```python
from build123d import *

# Parameters (mm, degrees)
F1_DEPTH  = 127
F2_R      = 104.325393
F2_R_2    = 26.179728
F2_R_3    = 10.594913
F3_DEPTH  = 38.1
F3_FACE_R = 10.594913
F4_DEPTH  = 38.1
F5_R      = 9.525
F6_DEPTH  = 127


with BuildPart() as f1:
    # F0 (on Front) → F1 (new body)
    with BuildSketch(Plane.XZ):
        Polygon((12.158688, 37.641967), (-25.941312, 37.641967), (-25.941312, -13.158033), (-16.416312, -13.158033), (-16.416312, -25.858033), (2.62328, -25.858033), (2.62328, -13.26213), (12.158688, -13.26213), align=None)
    extrude(amount=F1_DEPTH)

    # F2 (on Right) → F3 (cut)
    with BuildSketch(Plane.YZ):
        with Locations((-442.556002, 14.38355)):
            Circle(F2_R)
        with Locations((196.325033, 10.431935)):
            Circle(F2_R_2)
        with Locations((-94.180087, 11.172054)):
            Circle(F2_R_3)
        with Locations((-32.819913, 11.172054)):
            Circle(F2_R_3)
    extrude(amount=-F3_DEPTH, mode=Mode.SUBTRACT)

    # F3_face (on face) → F4 (cut)
    with BuildSketch(Plane(origin=(0, -32.819913, 11.172054), x_dir=(0, 1, 0), z_dir=(-1, 0, 0))):
        Circle(F3_FACE_R)
        with Locations((-61.360174, 0)):
            Circle(F3_FACE_R)
    extrude(amount=-F4_DEPTH, mode=Mode.SUBTRACT)

    # F5 (on Front) → F6 (cut)
    with BuildSketch(Plane.XZ):
        with Locations((-6.891312, 12.241967)):
            Circle(F5_R)
    extrude(amount=F6_DEPTH, mode=Mode.SUBTRACT)


solid = f1.part
```
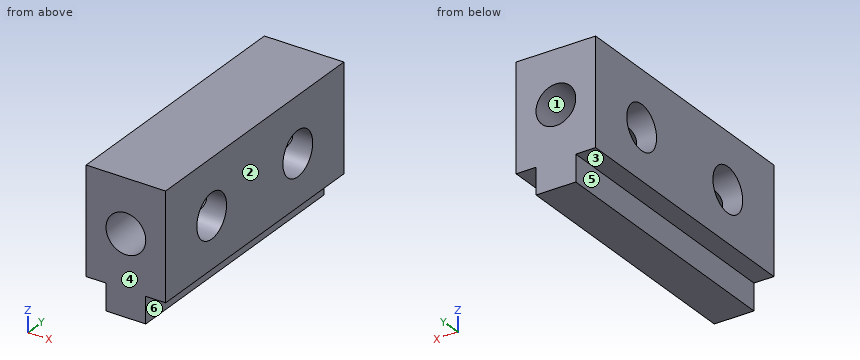
Geometry check sheet. Reference: the model listing, model coordinates, mm. Face numbers are marked on the shaded views. A direction names the side the tool comes from. Coordinates: 2 decimals unless noted, no trailing zeros. Write each loop counter-clockwise with the first axis right and the second up, starting at its lowest first coordinate (ties: lowest second). Pieces come first, ordered by that corner, then holes. Notation, with made-up numbers: (57, 36) -> (89, 36) arc R9 cw to (89, 46) -> close; hole circle Ø2 at (75.25, 85.5). An arc over 180 degrees is marked (long way). Use CSV: the item, a comma, the result in double quotes. Start each with the question number.
Item 1: Set-up check for the marked faces 4, 5 and 6: record each of +Z, -Z, +X, -X, +Y, -Y from which the full face is reachable in a straight line by a thin tool's end or side.
Item 2: Cross-section at B-B, the plane y = -41. Record the cut outline in (x, z) (3 decimals).
Item 3: Cross-section at A-A, the plane x = -4. Record the cut outline in (y, z).
Item 4: Cross-section at D-D, the plane y = -57.5. Record the cut outline in (x, z) (3 decimals), plus the area to 3 significant figures.
Item 5: Cross-section at C-C, the plane z = 18. Record the cut outline in (x, y), plus the area to 3 significant figures.
Item 6: Thickness scan on line 1 (Y direction, x = -23.5, z = 6); line 2 (Z direction, x = -7, y = -45.5); line 3 (Z direction, x = -7.5, y = -19.5). Record the ranges inside material, lowest first.
Item 7: Mould release check, pull along X, two halves, no side actions. Record for the marked faces 1, 2 and 3: released by +X, released by -X, zero draft, split by the parting line, or undercut.
Item 8: Depth check by flat-ended pin: pin 1 Ø3 at (x, y) = (-20.5, -87) entering from -Z; pin 2 Ø10 at (y, z) = (-44, -19.5) entering from +X; pin 3 Ø6.5 at (y, z) = (-50.5, -17) entering from -X. Enter the tip coordinate at first touch or a pass-through.
Answers:
1,face 4,"+Z, -Z, +X, -X, -Y"
1,face 5,"-Z, -X, +Y, -Y"
1,face 6,"-Z, +X, +Y, -Y"
2,outline,"(-25.941, -13.158) -> (-16.416, -13.158) -> (-16.416, -25.858) -> (2.623, -25.858) -> (2.623, -13.262) -> (12.159, -13.262) -> (12.159, 4.439) -> (-1.429, 4.439) arc R9.525 cw to (-12.353, 4.439) -> (-25.941, 4.439) -> close; (-25.941, 17.905) -> (-14.55, 17.905) arc R9.525 cw to (0.767, 17.905) -> (12.159, 17.905) -> (12.159, 37.642) -> (-25.941, 37.642) -> close"
3,outline,"(-127, -25.86) -> (0, -25.86) -> (0, 3.17) -> (-25.88, 3.17) arc R10.59 cw to (-39.76, 3.17) -> (-87.24, 3.17) arc R10.59 cw to (-101.12, 3.17) -> (-127, 3.17) -> close; (-127, 21.32) -> (-97.23, 21.32) arc R10.59 cw to (-91.13, 21.32) -> (-35.87, 21.32) arc R10.59 cw to (-29.77, 21.32) -> (0, 21.32) -> (0, 37.64) -> (-127, 37.64) -> close"
4,outline,"(-25.941, -13.158) -> (-16.416, -13.158) -> (-16.416, -25.858) -> (2.623, -25.858) -> (2.623, -13.262) -> (12.159, -13.262) -> (12.159, 37.642) -> (-25.941, 37.642) -> close; hole circle Ø19.05 at (-6.891, 12.242)"
4,area,"1,890 mm^2"
5,outline,"(-25.94, -127) -> (-14.48, -127) -> (-14.48, -102.28) -> (-25.94, -102.28) -> close; (-25.94, -86.08) -> (-14.48, -86.08) -> (-14.48, -40.92) -> (-25.94, -40.92) -> close; (-25.94, -24.72) -> (-14.48, -24.72) -> (-14.48, 0) -> (-25.94, 0) -> close; (0.7, -127) -> (12.16, -127) -> (12.16, -102.28) -> (0.7, -102.28) -> close; (0.7, -86.08) -> (12.16, -86.08) -> (12.16, -40.92) -> (0.7, -40.92) -> close; (0.7, -24.72) -> (12.16, -24.72) -> (12.16, 0) -> (0.7, 0) -> close"
5,area,"2,170 mm^2"
6,line 1,"-127 to -103.43, -84.93 to -42.07, -23.57 to 0"
6,line 2,"-25.86 to 2.72, 21.77 to 37.64"
6,line 3,"-25.86 to 2.74, 21.75 to 37.64"
7,face 1,"undercut"
7,face 2,"released by +X"
7,face 3,"zero draft"
8,pin 1,"z = -13.16"
8,pin 2,"x = 2.62"
8,pin 3,"x = -16.42"
